Part model, mm, in its own coordinate system. Coordinates: 2 decimals unless noted, no trailing zeros. Loops run counter-clockwise (first coordinate to the right, second up) from the corner with the lowest first, then second, coordinate; pieces in that order, holes last. Notation, with made-up numbers: (61, 10.5) - (97, 10.5) arc R30 cw to (97, 47.5) - close; hole circle Ø2 at (16.5, 26.25). An arc over 180 degrees is marked (long way). Use a Markdown table: item, result. Add a question column.
1) Probe probe 1 along Y at (x, z) = (11.5, 0.45); probe 2 along Y at (x, z) = (10, 0.9); probe 3 along X at (y, z) = (9.5, 0.6). List the from-to ranges inside material, lowest first. Write a range as [from, to].
2) Band-saw the part on B-B (x = 8.75). Give the cut face in (y, z) (3 decimals).
3) Band-saw the part on C-C (y = 31). Give the cut face in (x, z) (3 decimals), plus the area to 3 significant figures.
4) Band-saw the part on A-A (z = 2.9). Give the cut face in (x, y).
Autodesk Inventor part; units mm, degrees
ref_plane "YZ Plane" through (0, 0, 0) normal (1, 0, 0) x (0, 1, 0)
ref_plane "XZ Plane" through (0, 0, 0) normal (0, 1, 0) x (-1, 0, 0)
ref_plane "XY Plane" through (0, 0, 0) normal (0, 0, 1) x (1, 0, 0)
sketch "Sketch1" plane through (0, 0, 0) normal (0, 0, 1) x (1, 0, 0)
  line L0 (21.6079, 10.4672) -> (13.9879, 6.0678)
  line L1 (13.9879, 6.0678) -> (6.3679, 10.4672)
  line L2 (6.3679, 29.8109) -> (13.9879, 34.2103)
  line L3 (13.9879, 34.2103) -> (21.6079, 29.8109)
  line L4 (6.3679, 29.8109) -> (6.3679, 10.4672)
  line L5 (21.6079, 29.8109) -> (21.6079, 10.4672)
  point P0 (0, 0)
  point P1 (13.9879, 20.1391)
  dimension "d2" = 28.1426
  dimension "d3" = 15.24
extrude "Extrusion1" add sketch "Sketch1" along normal blind 3.175
sketch "Sketch2" plane through (0, 0, 3.175) normal (0, 0, 1) x (1, 0, 0)
  line L0 (7.1627, 16.7783) -> (25.4618, 16.7783) construction
  line L1 (25.4618, 16.7783) -> (25.4618, 11.2346) construction
  line L2 (25.4618, 11.2346) -> (7.1627, 11.2346) construction
  line L3 (7.1627, 11.2346) -> (7.1627, 16.7783) construction
  point P0 (0, 0)
properties part number "Academies logo"
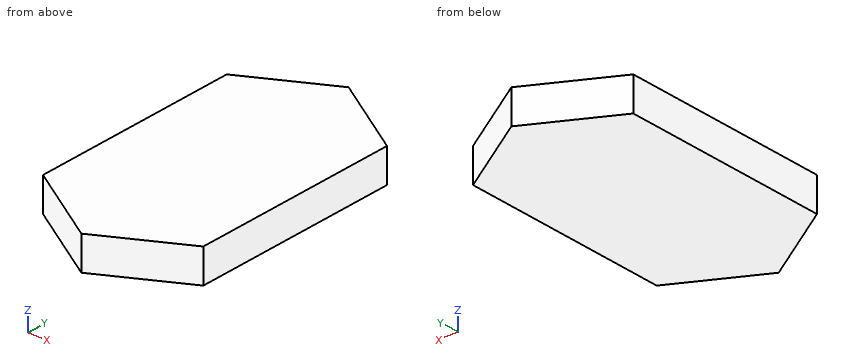
Answer block:
| question | item | result |
|---|---|---|
| 1 | probe 1 | [7.5, 32.77] |
| 1 | probe 2 | [8.37, 31.91] |
| 1 | probe 3 | [8.04, 19.93] |
| 2 | outline | (9.092, 0) - (31.186, 0) - (31.186, 3.175) - (9.092, 3.175) - close |
| 3 | outline | (8.427, 0) - (19.548, 0) - (19.548, 3.175) - (8.427, 3.175) - close |
| 3 | area | 35.3 mm2 |
| 4 | outline | (6.37, 10.47) - (13.99, 6.07) - (21.61, 10.47) - (21.61, 29.81) - (13.99, 34.21) - (6.37, 29.81) - close |
